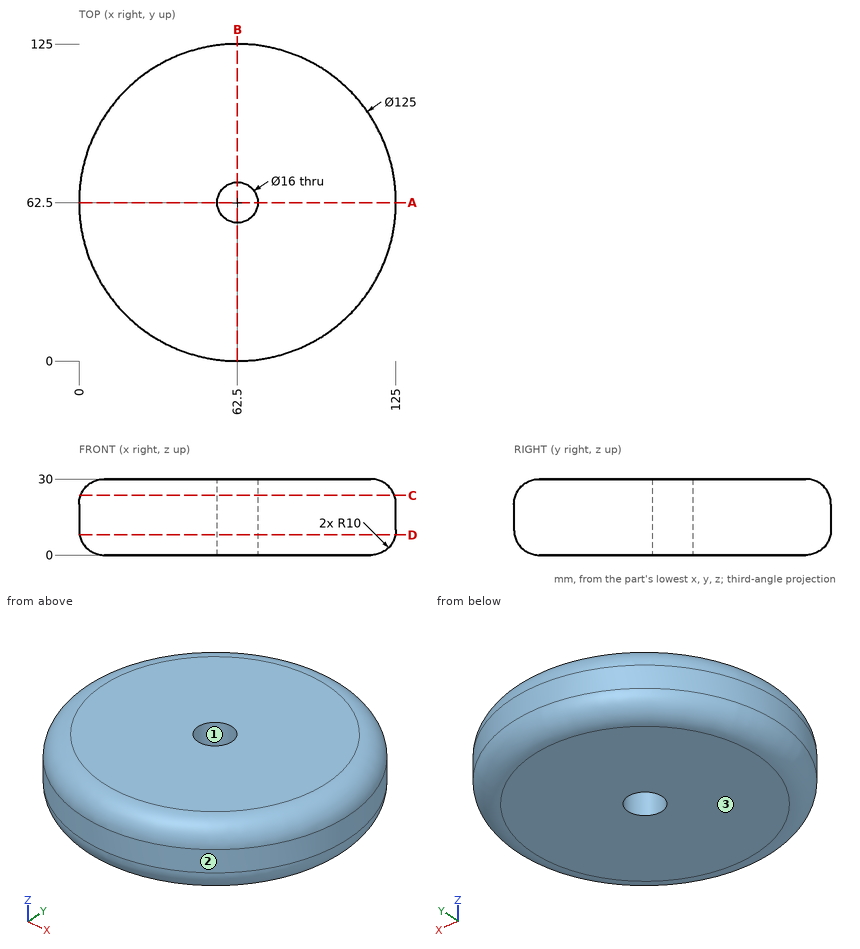
Check sheet for the drawn part. Datum: minimum x, y, z corner. Units: mm. Round coordinates to 2 decimals unless told otherwise and drop trailing zeros. Write each loop counter-clockwise with the first axis right and the second up, starting at its lowest first coordinate (ties: lowest second). Pieces come first, ordered by that corner, then holes. Notation, with made-up numbers: (15.5, -2.5) -> (27.5, -2.5) arc R28 ccw to (27.5, 25.5) -> close; hole circle Ø8 at (30, -29). An arc over 180 degrees is marked (long way). Write each question's results on one line, items separated by ' | '.
Q1. Thickness scan on probe 1 along Y at (x, z) = (62.5, 16.25); probe 2 along Y at (x, z) = (56, 15); probe 3 along X at (y, z) = (57, 23.5). Record the ranges inside material, lowest first.
Derived:
probe 1: y = 0 to 54.5, 70.5 to 125 | probe 2: y = 0.34 to 57.84, 67.16 to 124.66 | probe 3: x = 0.88 to 56.69, 68.31 to 124.12
Q2. Sectioned sample at D-D, the plane z = 8. Record the boundary of the cut face in (x, y), and give its area (3 significant figures).
Derived:
outline: circle Ø124.6 at (62.5, 62.5); hole circle Ø16 at (62.5, 62.5) | area: 12,000 mm²
Q3. Sectioned sample at A-A, the plane y = 62.5. Record the boundary of the cut face in (x, z).
Derived:
outline: (0, 10) arc R10 ccw to (10, 0) -> (54.5, 0) -> (54.5, 30) -> (10, 30) arc R10 ccw to (0, 20) -> close; (70.5, 0) -> (115, 0) arc R10 ccw to (125, 10) -> (125, 20) arc R10 ccw to (115, 30) -> (70.5, 30) -> close
Q4. Draft check along Y on the marked faces 1, 2 and 3. Enter one of: released by +Y, released by -Y, zero draft, split by the parting line, or undercut.
Derived:
face 1: undercut | face 2: split by the parting line | face 3: zero draft
Q5. Go/stop test with flat-tipped pins: pin 1 Ø1.5 at (y, z) = (27, 8) entering from +X; pin 2 Ø10 at (x, z) = (13.5, 25.5) entering from +Y; pin 3 Ø4 at (x, z) = (100, 25) entering from +Y. Record where each tip stops, or that it passes through.
Derived:
pin 1: stops at x = 114.23 | pin 2: stops at y = 105.57 | pin 3: stops at y = 112.74
Q6. Sectioned sample at C-C, the plane z = 23.5. Record the boundary of the cut face in (x, y) (1 decimal), and give its area (3 significant figures).
Derived:
outline: circle Ø123.7 at (62.5, 62.5); hole circle Ø16 at (62.5, 62.5) | area: 11,800 mm²
